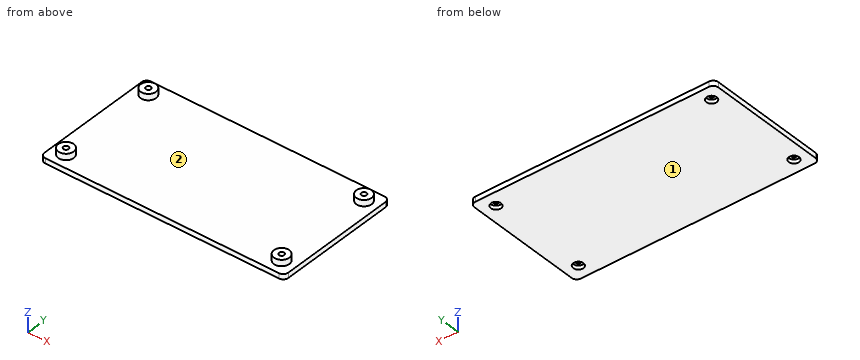
from build123d import *

# Parameters (mm, degrees)
SKETCH_1_W          = 95
SKETCH_1_H          = 50
EXTRUDE_1_DEPTH     = 2
EXTRUDE_START       = -2
SKETCH_3_R          = 3
EXTRUDE_3_DEPTH     = 2.4
SKETCH_4_R          = 2
CUT_EXTRUDE_1_DEPTH = 1.5
SKETCH_5_R          = 1
CUT_EXTRUDE_2_DEPTH = 54.857311481
FILLET_2_R          = 2


with BuildPart() as part:
    # 草图1 → 凸台-拉伸1 (new body)
    with BuildSketch(Plane.XY):
        Rectangle(SKETCH_1_W, SKETCH_1_H)
    extrude(amount=EXTRUDE_1_DEPTH)

    # 草图3 → 凸台-拉伸3 (add)
    with BuildSketch(Plane(origin=(0, 0, 0), x_dir=(-1, 0, 0), z_dir=(0, 0, -1)).offset(EXTRUDE_START)):
        with Locations((-42, 19.50009906)):
            Circle(SKETCH_3_R)
        with Locations((42.00021336, 19.50009906)):
            Circle(SKETCH_3_R)
        with Locations((42.00021336, -19.5)):
            Circle(SKETCH_3_R)
        with Locations((-42, -19.5)):
            Circle(SKETCH_3_R)
    extrude(amount=-EXTRUDE_3_DEPTH)

    # 草图4 → 切除-拉伸1 (cut)
    with BuildSketch(Plane(origin=(0, 0, 0), x_dir=(-1, 0, 0), z_dir=(0, 0, -1))):
        with Locations((-42, 19.50009906)):
            Circle(SKETCH_4_R)
        with Locations((-42, -19.5)):
            Circle(SKETCH_4_R)
        with Locations((42.00021336, 19.50009906)):
            Circle(SKETCH_4_R)
        with Locations((42.00021336, -19.5)):
            Circle(SKETCH_4_R)
    extrude(amount=-CUT_EXTRUDE_1_DEPTH, mode=Mode.SUBTRACT)

    # 草图5 → 切除-拉伸2 (cut, through all)
    with BuildSketch(Plane(origin=(0, 0, 0), x_dir=(-1, 0, 0), z_dir=(0, 0, -1))):
        with Locations((-42, 19.50009906)):
            Circle(SKETCH_5_R)
        with Locations((42.00021336, 19.50009906)):
            Circle(SKETCH_5_R)
        with Locations((42.00021336, -19.5)):
            Circle(SKETCH_5_R)
        with Locations((-42, -19.5)):
            Circle(SKETCH_5_R)
    extrude(amount=-CUT_EXTRUDE_2_DEPTH, mode=Mode.SUBTRACT)

    # 圆角2
    fillet_2_edges = [part.edges().sort_by_distance(p)[0] for p in [
        (47.5, -25, 1),
        (-47.5, -25, 1),
        (-47.5, 25, 1),
        (47.5, 25, 1),
    ]]
    fillet(fillet_2_edges, radius=FILLET_2_R)


solid = part.part
Can you work these out from the model? Positions are in its coordinate system, mm. Face numbers are marked on the shaded views. Coordinates: 2 decimals unless noted, no trailing zeros. Order: outer loops, then holes, each group sorted by start corner. A loop starts at its lowest first (then second) coordinate and runs counter-clockwise, first axis right, second up. Notation, with made-up numbers: (77.5, 60) - (85.5, 60) arc R27 cw to (85.5, 80) - close; hole circle Ø11 at (70.5, -5.5). An arc over 180 degrees is marked (long way). Answer as a JSON object with one key per item and string values. Group by question number.
Q1. Imagine slicing it at A-A (y = -19.5). Please give me the cut outline in (x, z).
Q2. I need wall thicknesses on line 1 (Y direction, x = 42, z = 0.65); line 2 (X direction, y = -19, z = 2.3); line 3 (Z direction, x = -2.5, y = -4.5). Which ranges of each line are inside material? Lowest first, please. Write a range as from..to.
Q3. Imagine slicing it at C-C (x = 42). Please give me the cut outline in (y, z), and give its area (3 significant figures).
Q4. We'd pull the mould along X, two halves only. Please class the marked faces 1 and 2: +X half, -X half, draft (parallel to the pull), parting line (faces both ways), or undercut.
Q5. Will these pins go through, and if not, where does the flat tip stop? P1, Ø3, axis at x = 42, y = -19.5, coming from the -Z side; P2, Ø5, axis at x = -12, y = -1.5, coming from the +Z side.
Q6. Imagine slicing it at B-B (z = 2.75). Please give me the cut outline in (x, y), and give its area (3 significant figures).
Q7. Imagine slicing it at D-D (y = 13). Please give me the cut outline in (x, z).
Determined:
{
 "1": {"outline": "(-47.5, 0) - (-44, 0) - (-44, 1.5) - (-43, 1.5) - (-43, 4.4) - (-45, 4.4) - (-45, 2) - (-47.5, 2) - close; (-41, 1.5) - (-40, 1.5) - (-40, 0) - (40, 0) - (40, 1.5) - (41, 1.5) - (41, 4.4) - (39, 4.4) - (39, 2) - (-39, 2) - (-39, 4.4) - (-41, 4.4) - close; (43, 1.5) - (44, 1.5) - (44, 0) - (47.5, 0) - (47.5, 2) - (45, 2) - (45, 4.4) - (43, 4.4) - close"},
 "2": {"line 1": "y = -25..-21.5, -17.5..17.5, 21.5..25", "line 2": "x = -44.96..-42.87, -41.13..-39.04, 39.04..41.13, 42.87..44.96", "line 3": "z = 0..2"},
 "3": {"outline": "(-25, 0) - (-21.5, 0) - (-21.5, 1.5) - (-20.5, 1.5) - (-20.5, 4.4) - (-22.5, 4.4) - (-22.5, 2) - (-25, 2) - close; (-18.5, 1.5) - (-17.5, 1.5) - (-17.5, 0) - (17.5, 0) - (17.5, 1.5) - (18.5, 1.5) - (18.5, 4.4) - (16.5, 4.4) - (16.5, 2) - (-16.5, 2) - (-16.5, 4.4) - (-18.5, 4.4) - close; (20.5, 1.5) - (21.5, 1.5) - (21.5, 0) - (25, 0) - (25, 2) - (22.5, 2) - (22.5, 4.4) - (20.5, 4.4) - close", "area": "105 mm2"},
 "4": {"face 1": "draft", "face 2": "undercut"},
 "5": {"P1": "stops at z = 1.5", "P2": "stops at z = 2"},
 "6": {"outline": "circle Ø6 at (-42, -19.5); circle Ø6 at (-42, 19.5); circle Ø6 at (42, -19.5); circle Ø6 at (42, 19.5); hole circle Ø2 at (-42, -19.5); hole circle Ø2 at (-42, 19.5); hole circle Ø2 at (42, -19.5); hole circle Ø2 at (42, 19.5)", "area": "101 mm2"},
 "7": {"outline": "(-47.5, 0) - (47.5, 0) - (47.5, 2) - (-47.5, 2) - close"}
}
